Check sheet for the modelled part. Datum: model origin and axes. Units: mm. Face numbers are marked on the shaded views. A direction names the side the tool comes from. Round coordinates to 2 decimals unless told otherwise and drop trailing zeros. Write each loop counter-clockwise with the first axis right and the second up, starting at its lowest first coordinate (ties: lowest second). Pieces come first, ordered by that corner, then holes. Notation, with made-up numbers: (12, 52.25) -> (64, 52.25) arc R16 cw to (64, 78.25) -> close; hole circle Ø10 at (40.5, 36). An arc over 180 degrees is marked (long way). Answer as a JSON object with one key per item and string values. Group by question number.
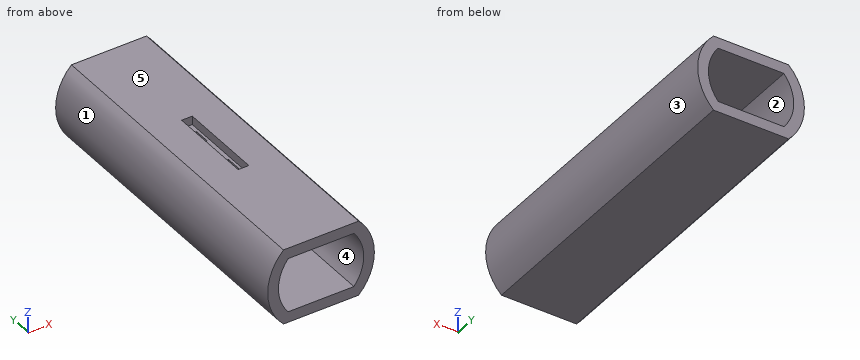
```python
from build123d import *

# Parameters (mm, degrees)
F1_DEPTH = 300
F3_DEPTH = 300
F4_W     = 10
F4_H     = 80
F5_DEPTH = 8
F6_W     = 5
F6_H     = 15
F7_DEPTH = 5


with BuildPart() as f1:
    # F0 (on Front) → F1 (new body)
    with BuildSketch(Plane.XZ):
        with BuildLine():
            Line((35.210084, 35.5), (-35.210084, 35.5))
            ThreePointArc((-35.210084, 35.5), (-50, 0), (-35.210084, -35.5))
            Line((-35.210084, -35.5), (35.210084, -35.5))
            ThreePointArc((35.210084, -35.5), (50, 0), (35.210084, 35.5))
        make_face()
    extrude(amount=F1_DEPTH)

    # F2 (on face) → F3 (cut)
    with BuildSketch(Plane.XZ.offset(300)):
        with BuildLine():
            Line((30.818014, 25.5), (-30.818014, 25.5))
            ThreePointArc((-30.818014, 25.5), (-40, 0), (-30.818014, -25.5))
            Line((-30.818014, -25.5), (30.818014, -25.5))
            ThreePointArc((30.818014, -25.5), (40, 0), (30.818014, 25.5))
        make_face()
    extrude(amount=-F3_DEPTH, mode=Mode.SUBTRACT)

    # F4 (on face) → F5 (cut)
    with BuildSketch(Plane.XY.offset(35.5)):
        with Locations((0.210084, -150)):
            Rectangle(F4_W, F4_H)
    extrude(amount=-F5_DEPTH, mode=Mode.SUBTRACT)

    # F6 (on face) → F7 (cut)
    with BuildSketch(Plane.XY.offset(27.5)):
        with Locations((0.210084, -127.5)):
            Rectangle(F6_W, F6_H)
        with Locations((0.210084, -172.5)):
            Rectangle(F6_W, F6_H)
    extrude(amount=-F7_DEPTH, mode=Mode.SUBTRACT)


solid = f1.part
```
(1) Section check B-B on z = -0.5. Record the cut outline in (x, y), then the cut area to 3 significant figures.
(2) Access from +Z, -Z, +X, -X, +Y, -Y to the whole of each face (thin tool, end or side, straight path). Record for the marked faces 1 and 2.
(3) Release check for a two-part mould opening along Z. For the marked faces 3, 4 and 5 record: pulls with the +Z half, pulls with the -Z half, needs draft (parallel to the pull), parting line crosses it, or undercut.
(4) Section check C-C on y = -125. Record the cut outline in (x, z), then the cut area to 3 significant figures.
(5) Section check A-A on x = 9. Record the cut outline in (y, z), then the cut area to 3 significant figures.
(6) Section check D-D on y = -243. Record the cut outline in (x, z), then the cut area to 3 significant figures.
(7) Go/stop test with flat-tipped pins: pin 1 Ø2.5 at (y, z) = (-132.5, 30.5) entering from -X; pin 2 Ø0.6 at (y, z) = (-130.5, 26.5) entering from +X; pin 3 Ø4 at (y, z) = (-85.5, 12) entering from +X. Record where each tip stops, or that it passes through.
(8) Scan lines: line 1 along X through (y, z) = (-243.5, -0.5); line 2 along Z through (x, y) = (10.5, -75); line 3 along Z through (x, y) = (-3, -153). Record each from-to range of solid material in increasing order.
Data:
{
 "1": {"outline": "(-50, -300) -> (-40, -300) -> (-40, 0) -> (-50, 0) -> close; (40, -300) -> (50, -300) -> (50, 0) -> (40, 0) -> close", "area": "6,000 mm²"},
 "2": {"face 1": "-X, +Y, -Y", "face 2": "+Y, -Y"},
 "3": {"face 3": "parting line crosses it", "face 4": "undercut", "face 5": "pulls with the +Z half"},
 "4": {"outline": "(-35.21, -35.5) -> (35.21, -35.5) arc R50 ccw to (35.21, 35.5) -> (5.21, 35.5) -> (5.21, 27.5) -> (2.71, 27.5) -> (2.71, 25.5) -> (30.82, 25.5) arc R40 cw to (30.82, -25.5) -> (-30.82, -25.5) arc R40 cw to (-30.82, 25.5) -> (-2.29, 25.5) -> (-2.29, 27.5) -> (-4.79, 27.5) -> (-4.79, 35.5) -> (-35.21, 35.5) arc R50 ccw to start", "area": "2,570 mm²"},
 "5": {"outline": "(-300, -35.5) -> (0, -35.5) -> (0, -25.5) -> (-300, -25.5) -> close; (-300, 25.5) -> (0, 25.5) -> (0, 35.5) -> (-300, 35.5) -> close", "area": "6,000 mm²"},
 "6": {"outline": "(-35.21, -35.5) -> (35.21, -35.5) arc R50 ccw to (35.21, 35.5) -> (-35.21, 35.5) arc R50 ccw to start; hole (-30.82, -25.5) -> (30.82, -25.5) arc R40 ccw to (30.82, 25.5) -> (-30.82, 25.5) arc R40 ccw to start", "area": "2,660 mm²"},
 "7": {"pin 1": "stops at x = -40.55", "pin 2": "stops at x = 42.59", "pin 3": "stops at x = 48.99"},
 "8": {"line 1": "x = -50 to -40, 40 to 50", "line 2": "z = -35.5 to -25.5, 25.5 to 35.5", "line 3": "z = -35.5 to -25.5, 25.5 to 27.5"}
}
